Can you work these out from the model? Positions are in its coordinate system, mm. A direction names the side the tool comes from. Coordinates: 2 decimals unless noted, no trailing zeros. Loops run counter-clockwise (first coordinate to the right, second up) from the corner with the lowest first, then second, coordinate; pieces in that order, holes last. Notation, with made-up numbers: M -3.75,67 L 28.25,67 A21 cw 28.25,76 Z; hole C -14,56 d6. An arc over 180 degrees is marked long. Return JSON: item names as keys, results as strings. Group by question number.
```python
from build123d import *

# Parameters (mm, degrees)
BOSS_EXTRUDE1_DEPTH = 76.2
SKETCH6_W           = 6.35
SKETCH6_H           = 31.75
CUT_EXTRUDE2_DEPTH  = 25.4
FILLET2_R           = 0.8128
SKETCH7_R           = 6.35
CUT_EXTRUDE3_DEPTH  = 76.2
CHAMFER1_SIZE       = 1.524
SKETCH8_W           = 6.35
SKETCH8_H           = 31.75
CUT_EXTRUDE4_DEPTH  = 125.609544076
FILLET3_R           = 0.8128


with BuildPart() as part:
    # Sketch2 → Boss-Extrude1 (new body)
    with BuildSketch(Plane.XY):
        Polygon((-62.567231638, 49.006214689), (-62.567231638, -14.493785311), (-24.467231638, -52.593785311), (26.332768362, -52.593785311), (26.332768362, -27.193785311), (7.282768362, -27.193785311), (7.282768362, -1.793785311), (-18.117231638, 23.606214689), (-37.167231638, 23.606214689), (-37.167231638, 49.006214689), align=None)
    extrude(amount=-BOSS_EXTRUDE1_DEPTH)

    # Sketch6 → Cut-Extrude2 (cut)
    with BuildSketch(Plane(origin=(0, 49.006214689, 0), x_dir=(1, 0, 0), z_dir=(0, 1, 0))):
        with Locations((-40.342231638, 38.1)):
            Rectangle(SKETCH6_W, SKETCH6_H)
    extrude(amount=-CUT_EXTRUDE2_DEPTH, mode=Mode.SUBTRACT)

    # Fillet2
    fillet2_edges = [part.edges().sort_by_distance(p)[0] for p in [
        (-43.517231638, 36.306214689, -22.225),
        (-43.517231638, 36.306214689, -53.975),
    ]]
    fillet(fillet2_edges, radius=FILLET2_R)

    # Sketch7 → Cut-Extrude3 (cut)
    with BuildSketch(Plane(origin=(2.744491525, 2.744491525, 0), x_dir=(0, 0, -1), z_dir=(0.7071067811865436, 0.7071067811865515, 0))):
        with Locations(Location((57.15, 11.539707349, 0), (0, 0, 90))):
            Circle(SKETCH7_R)
        with Locations(Location((19.05, 11.539707349, 0), (0, 0, 90))):
            Circle(SKETCH7_R)
    extrude(amount=-CUT_EXTRUDE3_DEPTH, mode=Mode.SUBTRACT)

    # Chamfer1
    chamfer1_edges = [part.edges().sort_by_distance(p)[0] for p in [
        (-0.925185733, 6.414168784, -19.05),
        (-0.925185733, 6.414168784, -57.15),
    ]]
    chamfer(chamfer1_edges, length=CHAMFER1_SIZE)

    # Sketch8 → Cut-Extrude4 (cut, through all)
    with BuildSketch(Plane(origin=(0, -27.193785311, 0), x_dir=(1, 0, 0), z_dir=(0, 1, 0))):
        with Locations((23.157768362, 38.1)):
            Rectangle(SKETCH8_W, SKETCH8_H)
    extrude(amount=-CUT_EXTRUDE4_DEPTH, mode=Mode.SUBTRACT)

    # Fillet3
    fillet3_edges = [part.edges().sort_by_distance(p)[0] for p in [
        (19.982768362, -39.893785311, -22.225),
        (19.982768362, -39.893785311, -53.975),
    ]]
    fillet(fillet3_edges, radius=FILLET3_R)


solid = part.part
```
1) Suppose I cut it at D-D, the plane x = -15. Give the number of separate pieces and of enclosed holes in the cut face, then the cut area to 3 significant figures.
2) If I drill on line 1 (Z direction, x = -23, y = -8); line 2 (X direction, y = -10.5, z = -69.5); line 3 (Y direction, x = 10.5, z = -21), over which ranges is the centre line in solid material (lowest first)? Write a range as from..to.
3) For pin 1 (6.5 mm diameter, centred on y = 39, z = -11.5, fed in from +X); pin 2 (20.5 mm diameter, centred on y = 34.5, z = -36, fed in from +X); pin 3 (4 mm diameter, centred on y = -28, z = -66, fed in from -X), each with a flat end and sliding along its axis, tell me the tip position at first contact or that it passes through.
4) Suppose I cut it at C-C, the plane x = 14. List the corners of the cut face in (y, z) for me.
5) If we mould it in two halves opening along Z, with no side actions, what happens to faces 4 (the face through (-29, -12, 0)), 5 (the face through (24, -40, -53.975)), 6 (the face through (-62.567, 18, -38))? For each: +Z half, -Z half, draft (parallel to the pull), parting line (faces both ways), or undercut.
6) Suppose I cut it at A-A, the plane y = 38. List the corners of the cut face in (x, z) for me (3 decimals).
7) Suppose I cut it at B-B, the plane z = -71. List the corners of the cut face in (x, y) for me.
8) For faces 1 (the face through (-40, 36, -22.225)), 2 (the face through (17, -27.194, -38)), 3 (the face through (19.983, -40, -38)), which set-ups out of +Z, -Z, +X, -X, +Y, -Y let a thin tool reach every point of the face, with its end or its side?
Returned:
{
 "1": {"separate pieces": "1", "enclosed holes": "2", "area": "5,210 mm²"},
 "2": {"line 1": "z = -76.2..-63.43, -50.87..-25.33, -12.77..0", "line 2": "x = -62.57..7.28", "line 3": "y = -52.59..-27.19"},
 "3": {"pin 1": "stops at x = -37.17", "pin 2": "stops at x = -43.52", "pin 3": "stops at x = -51.06"},
 "4": {"outline": "M -52.59,-76.2 L -27.19,-76.2 L -27.19,0 L -52.59,0 Z"},
 "5": {"face 4": "+Z half", "face 5": "undercut", "face 6": "draft"},
 "6": {"outline": "M -62.567,-76.2 L -37.167,-76.2 L -37.167,-53.975 L -42.704,-53.975 A0.813 cw -43.517,-53.162 L -43.517,-23.038 A0.813 cw -42.704,-22.225 L -37.167,-22.225 L -37.167,0 L -62.567,0 Z"},
 "7": {"outline": "M -62.57,-14.49 L -24.47,-52.59 L 26.33,-52.59 L 26.33,-27.19 L 7.28,-27.19 L 7.28,-1.79 L -18.12,23.61 L -37.17,23.61 L -37.17,49.01 L -62.57,49.01 Z"},
 "8": {"face 1": "+X, +Y", "face 2": "+Z, -Z, +X, +Y", "face 3": "+X, +Y, -Y"}
}
